```python
from build123d import *

# Parameters (mm, degrees)
F0_W     = 85
F0_H     = 45
F0_W_2   = 80
F0_H_2   = 40
F1_DEPTH = 3
F2_DEPTH = 26
F3_R     = 2
F4_R     = 5.75
F5_DEPTH = 3
F6_R     = 1.6
F7_DEPTH = 25


with BuildPart() as f1:
    # F0 (on Top) → F1 (new body)
    with BuildSketch(Plane.XY):
        Rectangle(F0_W, F0_H)
        Rectangle(F0_W_2, F0_H_2, mode=Mode.SUBTRACT)
        Rectangle(F0_W_2, F0_H_2)
    extrude(amount=F1_DEPTH)

    # F0 (on Top) → F2 (join)
    with BuildSketch(Plane.XY):
        Rectangle(F0_W, F0_H)
        Rectangle(F0_W_2, F0_H_2, mode=Mode.SUBTRACT)
    extrude(amount=F2_DEPTH)

    # F3
    f3_edges = [f1.edges().sort_by_distance(p)[0] for p in [
        (-42.5, -22.5, 13),
        (42.5, -22.5, 13),
        (-42.5, 22.5, 13),
        (42.5, 22.5, 13),
    ]]
    fillet(f3_edges, radius=F3_R)

    # F4 (on face) → F5 (cut, through all)
    with BuildSketch(Plane.XY.offset(3)):
        with Locations((32.25, 0)):
            Circle(F4_R)
    extrude(amount=-F5_DEPTH, mode=Mode.SUBTRACT)

    # F6 (on face) → F7 (cut)
    with BuildSketch(Plane(origin=(0, 0, 0), x_dir=(1, 0, 0), z_dir=(0, 0, -1))):
        with Locations((-35.962, -15.942)):
            Circle(F6_R)
        with Locations((-35.962, 15.942)):
            Circle(F6_R)
        with Locations((35.962, 15.942)):
            Circle(F6_R)
        with Locations((35.962, -15.942)):
            Circle(F6_R)
    extrude(amount=-F7_DEPTH, mode=Mode.SUBTRACT)


solid = f1.part
```
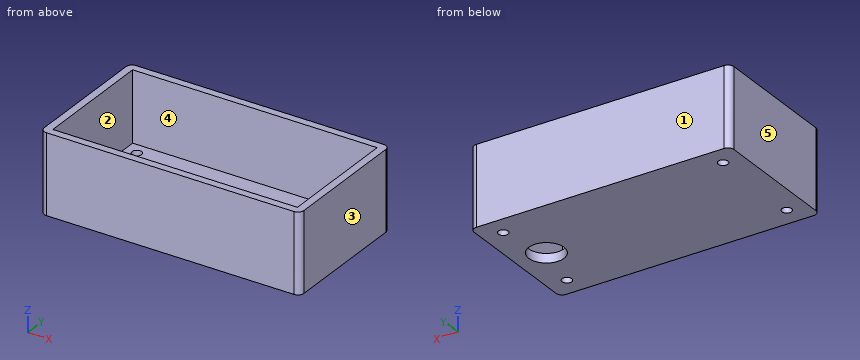
Build history of the part. All positions in model axes, mm. Face numbers are marked on the shaded views. A direction names the side the tool comes from. Coordinates: 2 decimals unless noted, no trailing zeros. Order: outer loops, then holes, each group sorted by start corner. A loop starts at its lowest first (then second) coordinate and runs counter-clockwise, first axis right, second up.
Item 1: Saw through at D-D on y = -11. List the corners of the cut face in (x, z).
Filled in:
outline: (-42.5, 0) - (42.5, 0) - (42.5, 26) - (40, 26) - (40, 3) - (-40, 3) - (-40, 26) - (-42.5, 26) - close
Item 2: Saw through at A-A on x = 32.25. List the corners of the cut face in (y, z).
Filled in:
outline: (-22.5, 0) - (-5.75, 0) - (-5.75, 3) - (-20, 3) - (-20, 26) - (-22.5, 26) - close; (5.75, 0) - (22.5, 0) - (22.5, 26) - (20, 26) - (20, 3) - (5.75, 3) - close
Item 3: Saw through at B-B on z = 7.75. List the corners of the cut face in (x, y).
Filled in:
outline: (-42.5, -20.5) arc R2 ccw to (-40.5, -22.5) - (40.5, -22.5) arc R2 ccw to (42.5, -20.5) - (42.5, 20.5) arc R2 ccw to (40.5, 22.5) - (-40.5, 22.5) arc R2 ccw to (-42.5, 20.5) - close; hole (-40, -20) - (40, -20) - (40, 20) - (-40, 20) - close
Item 4: Drop flat-ended pins along their axis: pin 1 Ø1.9 at (x, y) = (35.962, -15.942) entering from -Z; pin 2 Ø5 at (x, y) = (-12.5, 13) entering from +Z. Give the stop position or say it passes through.
Filled in:
pin 1: passes through
pin 2: stops at z = 3
Item 5: Tool access for the marked faces 4 and 5: list every direction of +Z, -Z, +X, -X, +Y, -Y with a clear straight run to the whole face (end or side of a thin tool).
Filled in:
face 4: +Z
face 5: +Z, -Z, -X, +Y, -Y
Item 6: Saw through at C-C on y = 0. List the corners of the cut face in (x, z).
Filled in:
outline: (-42.5, 0) - (26.5, 0) - (26.5, 3) - (-40, 3) - (-40, 26) - (-42.5, 26) - close; (38, 0) - (42.5, 0) - (42.5, 26) - (40, 26) - (40, 3) - (38, 3) - close
Item 7: Mould opens along X. For the marked faces 1, 2 and 3 say: released by +X, released by -X, zero draft, split by the parting line, or undercut.
Filled in:
face 1: zero draft
face 2: undercut
face 3: released by +X
Item 8: Drill centre lines: L1, parallel to Y at x = -11.5, z = 5.5; L2, parallel to X at y = -17.5, z = 8.5; L3, parallel to Z at x = -3.5, y = 19. Where is each one in solid material? Low to high.
Filled in:
L1: y = -22.5 to -20, 20 to 22.5
L2: x = -42.5 to -40, 40 to 42.5
L3: z = 0 to 3
